```python
from build123d import *

# Parameters (mm, degrees)
SKETCH1_W               = 20
SKETCH1_H               = 35
BOSS_EXTRUDE1_DEPTH     = 30
CHAMFER1_SIZE           = 25
FILLET1_R               = 1
SKETCH2_R               = 2.65
CUT_EXTRUDE2_DEPTH      = 20
SKETCH4_R               = 5.5
CUT_EXTRUDE3_DEPTH      = 20
SKETCH5_W               = 20.05
SKETCH5_H               = 6.8
CUT_EXTRUDE4_DEPTH      = 15
CUT_EXTRUDE5_DEPTH      = 6.8
FILLET3_R               = 1
SKETCH7_R               = 2.745697614
BOSS_EXTRUDE2_DEPTH     = 11
FILLET4_R               = 1
SKETCH10_R              = 1.65
CUT_EXTRUDE7_DEPTH      = 18
CUT_EXTRUDE8_DEPTH      = 8
CUT_EXTRUDE8_DEPTH_BACK = 8
SKETCH11_R              = 3


with BuildPart() as part:
    # Sketch1 → Boss-Extrude1 (new body)
    with BuildSketch(Plane(origin=(0, 0, 0), x_dir=(1, 0, 0), z_dir=(0, 1, 0))):
        Rectangle(SKETCH1_W, SKETCH1_H)
    extrude(amount=BOSS_EXTRUDE1_DEPTH)

    # Chamfer1
    chamfer1_edges = [part.edges().sort_by_distance(p)[0] for p in [
        (0, 30, 17.5),
    ]]
    chamfer(chamfer1_edges, length=CHAMFER1_SIZE)

    # Fillet1
    fillet1_edges = [part.edges().sort_by_distance(p)[0] for p in [
        (10, 30, -12.5),
        (0, 30, -7.5),
        (10, 2.5, 17.5),
        (10, 17.5, 5),
        (-10, 2.5, 17.5),
        (0, 5, 17.5),
        (0, 30, -17.5),
        (-10, 17.5, 5),
        (-10, 30, -12.5),
        (-10, 15, -17.5),
        (10, 15, -17.5),
    ]]
    fillet(fillet1_edges, radius=FILLET1_R)

    # Sketch2 → Cut-Extrude2 (cut)
    with BuildSketch(Plane(origin=(0, 0, 0), x_dir=(-1, 0, 0), z_dir=(0, -1, 0))):
        with Locations(Location((0, -7.5, 0), (0, 0, 90))):
            Circle(SKETCH2_R)
    extrude(amount=-CUT_EXTRUDE2_DEPTH, mode=Mode.SUBTRACT)

    # Sketch4 → Cut-Extrude3 (cut)
    with BuildSketch(Plane(origin=(0, 11, 0), x_dir=(-1, 0, 0), z_dir=(0, -1, 0))):
        with Locations((0, -7.5)):
            Circle(SKETCH4_R)
    extrude(amount=-CUT_EXTRUDE3_DEPTH, mode=Mode.SUBTRACT)

    # Sketch5 → Cut-Extrude4 (cut)
    with BuildSketch(Plane(origin=(0, 30, 0), x_dir=(1, 0, 0), z_dir=(0, 1, 0))):
        with Locations((1.516964354, 12.207106781)):
            Rectangle(SKETCH5_W, SKETCH5_H)
    extrude(amount=-CUT_EXTRUDE4_DEPTH, mode=Mode.SUBTRACT)

    # Sketch6 → Cut-Extrude5 (cut)
    with BuildSketch(Plane(origin=(0, 0, -8.807106781), x_dir=(-1, 0, 0), z_dir=(0, 0, -1))):
        with BuildLine():
            Line((-10, 10.37003714), (-10, 2.37003714))
            Line((-10, 2.37003714), (-5, 2.37003714))
            ThreePointArc((-5, 2.37003714), (1.70481367, 5.469731724), (4.254017823, 12.402565997))
            Line((4.254017823, 12.402565997), (4.254017823, 21.00909074))
            Line((4.254017823, 21.00909074), (-5.745982177, 21.00909074))
            Line((-5.745982177, 21.00909074), (-5.745982177, 14.664154296))
            ThreePointArc((-5.745982177, 14.664154296), (-6.989544506, 11.641898939), (-10, 10.37003714))
        make_face()
    extrude(amount=CUT_EXTRUDE5_DEPTH, mode=Mode.SUBTRACT)

    # Fillet3
    fillet3_edges = [part.edges().sort_by_distance(p)[0] for p in [
        (5.745982177, 15, -12.207106781),
        (-4.254017823, 15, -12.207106781),
    ]]
    fillet(fillet3_edges, radius=FILLET3_R)

    # Sketch7 → Boss-Extrude2 (add)
    with BuildSketch(Plane.XZ):
        with BuildLine():
            Line((7.5, -17.5), (-7.5, -17.5))
            Line((-7.5, -17.5), (-7.5, -27.5))
            ThreePointArc((-7.5, -27.5), (-6.328427125, -30.328427125), (-3.5, -31.5))
            Line((-3.5, -31.5), (3.5, -31.5))
            ThreePointArc((3.5, -31.5), (6.328427125, -30.328427125), (7.5, -27.5))
            Line((7.5, -27.5), (7.5, -17.5))
        make_face()
        with Locations(Location((0, -23.5, 0), (0, 0, 270))):
            Circle(SKETCH7_R, mode=Mode.SUBTRACT)
    extrude(amount=-BOSS_EXTRUDE2_DEPTH)

    # Fillet4
    fillet4_edges = [part.edges().sort_by_distance(p)[0] for p in [
        (6.328427125, 11, -30.328427125),
        (0, 11, -31.5),
        (-6.328427125, 11, -30.328427125),
        (-7.5, 11, -22.5),
        (7.5, 11, -22.5),
    ]]
    fillet(fillet4_edges, radius=FILLET4_R)

    # Sketch10 → Cut-Extrude7 (cut)
    with BuildSketch(Plane.XY.offset(-15.607106781)):
        with Locations(Location((-3.358035646, 22.55, 0), (0, 0, 90))):
            Circle(SKETCH10_R)
        with Locations(Location((6.341964354, 22.55, 0), (0, 0, 90))):
            Circle(SKETCH10_R)
    extrude(amount=CUT_EXTRUDE7_DEPTH, mode=Mode.SUBTRACT)

    # Sketch11 → Cut-Extrude8 (cut, two sides: drawn at the far end of the back side and taken through both)
    with BuildSketch(Plane(origin=(0, 0, 2.192893219), x_dir=(-1, 0, 0), z_dir=(0, 0, -1)).offset(-CUT_EXTRUDE8_DEPTH_BACK)):
        with Locations(Location((3.358035646, 22.55, 0), (0, 0, 227.566705352))):
            Circle(SKETCH11_R)
        with Locations(Location((-6.341964354, 22.55, 0), (0, 0, 207.623697814))):
            Circle(SKETCH11_R)
    extrude(amount=CUT_EXTRUDE8_DEPTH + CUT_EXTRUDE8_DEPTH_BACK, mode=Mode.SUBTRACT)


solid = part.part
```
Read the model definition and answer for the solid it produces. Units are mm, in the model's axes. A direction names the side the tool comes from. Round coordinates to 2 decimals unless told otherwise and drop trailing zeros. Write each loop counter-clockwise with the first axis right and the second up, starting at its lowest first coordinate (ties: lowest second). Pieces come first, ordered by that corner, then holes. Notation, with made-up numbers: (-27.5, 30) - (28.5, 30) arc R22 ccw to (28.5, 42) - close; hole circle Ø9 at (-29, 39.5). An arc over 180 degrees is marked (long way). One line per item, written item: value.
Q1. For a pull along X with two mould halves and no side action, classify faces 4 (the cylindrical face through (0, 15, 2)), 5 (the cylindrical face through (-7.199, 10.715, -22.57)), 6 (the flat face through (0, 18, -17.5)) as pulls with the +X half, pulls with the -X half, needs draft (parallel to the pull), parting line crosses it, or undercut.
The answers:
face 4: undercut
face 5: pulls with the -X half
face 6: needs draft
Q2. Find section A-A (z = -23.5). Determine the outline of the cut face in (x, y), and give its area (3 significant figures).
The answers:
outline: (-7.5, 0) - (-2.75, 0) - (-2.75, 11) - (-6.5, 11) arc R1 ccw to (-7.5, 10) - close; (2.75, 0) - (7.5, 0) - (7.5, 10) arc R1 ccw to (6.5, 11) - (2.75, 11) - close
area: 104 mm2
Q3. Which of the six approach directions +Z, -Z, +X, -X, +Y, -Y give full straight-line access (tool end or side, diameter ignored) to faces 1 (the flat face through (8.1, 23.1, -5.807)), 2 (the flat face through (7.5, 5, -23)), 3 (the flat face through (0.1, 11, 4.6))?
The answers:
face 1: +Z
face 2: -Z, +X, +Y, -Y
face 3: +Y
Q4. Find section B-B (y = 22.55). Count the separate pieces of the cut face and the enclosed holes in it, and give its area (3 significant figures).
The answers:
separate pieces: 3
enclosed holes: 0
area: 133 mm2
Q5. Straight lines are drawn through the part: line 1 (X direction, y = 22.55, z = -7.1); line 2 (X direction, y = 22.55, z = -4); line 3 (Z direction, x = 3.25, y = 26). For each, find the intervals that lie inside material, in ascending order. Write a range as from..to.
The answers:
line 1: x = -10..-5.01, -1.71..4.69, 7.99..10
line 2: x = -10..-6.36, -0.36..3.34, 9.34..10
line 3: z = -17.5..-15.61, -8.81..-3.5
Q6. Each of these flat-tipped pins is pushed along its axis until it touches: P1, Ø1, axis at x = 4.5, y = 25, coming from the +Z side; P2, Ø9, axis at x = 0, z = -23.5, coming from the +Y side; P3, Ø5, axis at y = 3, z = -22, coming from the +X side; P4, Ø3, axis at x = -1, z = -8.5, coming from the -Y side. Where does it stop, or does it pass through?
The answers:
P1: stops at z = -2.12
P2: stops at y = 11
P3: stops at x = 7.5
P4: stops at y = 0
